Autodesk Inventor part; units mm, degrees
ref_plane "YZ Plane" through (0, 0, 0) normal (1, 0, 0) x (0, 1, 0)
ref_plane "XZ Plane" through (0, 0, 0) normal (0, 1, 0) x (-1, 0, 0)
ref_plane "XY Plane" through (0, 0, 0) normal (0, 0, 1) x (1, 0, 0)
ref_plane "Plano de trabajo1" through (0, 0, 0) normal (0, 0, 1) x (1, 0, 0)
sketch "Boceto1" plane through (0, 0, 0) normal (0, 0, 1) x (1, 0, 0)
  circle A0 centre (18.3423, 0) radius 1.2028
  circle A1 centre (3.6423, 0) radius 1.2028
  circle A2 centre (10.9923, -7.35) radius 1.2028
  circle A3 centre (10.9923, 7.35) radius 1.2028
  circle A4 centre (10.9923, 0) radius 10.9823
  circle A5 centre (10.9923, 0) radius 2.7
  circle A6 centre (10.9923, 0) radius 12.5
  line L0 (10.9923, 0) -> (22.9923, 0)
  line L1 (10.9923, 0) -> (10.9923, 12.5)
  line L2 (10.9923, 12.5) -> (22.9923, 12.5)
  line L3 (10.9923, 0) -> (10.9923, -12.5)
  line L4 (10.9923, -12.5) -> (22.9923, -12.5)
  line L5 (22.9923, -12.5) -> (22.9923, 12.5)
  point P0 (0, 0)
  dimension "d0" = 25
  dimension "d1" = 12
  dimension "d2" = 12
extrude "Extrusión1" add sketch "Boceto1" along normal blind 3 contours L0 A4 L3 A2 A5 A0 | A0 L0 A5 L1 A3 A4 | L0 L5 A6 L3 A4 | A4 L1 A6 L5 L0 | L1 A3 A5 L3 A2 A4 | A4 L3 A6 L1 | L2 L5 A6 | A6 L5 L4
sketch "Boceto2" plane through (22.9923, -12.5, 0) normal (1, 0, 0) x (0, 0, -1)
  line L0 (0, 0) -> (0, 25)
  line L1 (0, 25) -> (-3, 25)
  line L2 (-3, 0) -> (-3, 25)
  line L3 (0, 0) -> (-3, 0)
  point P0 (0, 12.5)
extrude "Extrusión2" add sketch "Boceto2" along normal blind 8
sketch "Boceto3" plane through (0, 0, 0) normal (0, 0, -1) x (-1, 0, 0)
  line L0 (-10.9923, -12.5) -> (-30.9923, -12.5)
  arc A0 (-10.9923, -12.5) -> (-10.9923, 12.5) centre (-10.9923, 0) ccw
  line L1 (-10.9923, 12.5) -> (-30.9923, 12.5)
  line L2 (-30.9923, -12.5) -> (-30.9923, 12.5)
  circle A1 centre (-10.9923, 0) radius 2.7
  circle A2 centre (-10.9923, 7.35) radius 1.2028
  circle A3 centre (-18.3423, 0) radius 1.2028
  circle A4 centre (-3.6423, 0) radius 1.2028
  circle A5 centre (-10.9923, -7.35) radius 1.2028
  line L3 (-30.9923, 12.5) -> (-27.9923, 12.5)
  line L4 (-27.9923, 12.5) -> (-27.9923, -12.5)
  line L5 (-27.9923, -12.5) -> (-30.9923, -12.5)
  line L6 (-30.9923, -12.5) -> (-30.9923, 12.5)
  point P0 (0, 0)
  dimension "d7" = 3
extrude "Extrusión3" add sketch "Boceto3" along normal blind 42 contours L0 L2 L1 L4
sketch "Boceto4" plane through (27.9923, -12.5, 0) normal (-1, 0, 0) x (0, 0, 1)
  line L0 (-42, 0) -> (-42, 25)
  line L1 (0, 25) -> (0, 0)
  line L2 (0, 25) -> (-42, 25)
  line L3 (-42, 0) -> (-42, 25)
  line L4 (0, 0) -> (-42, 0)
  line L5 (-42, 0) -> (-40, 0)
  line L6 (-40, 0) -> (-40, 25)
  line L7 (-40, 25) -> (-42, 25)
  line L8 (-42, 25) -> (-42, 0)
  point P0 (0, 12.5)
  dimension "d10" = 2
extrude "Extrusión4" add sketch "Boceto4" along normal blind 30 contours L0 L2 L6 L4
sketch "Boceto5" plane through (0, 0, -42) normal (0, 0, -1) x (-1, 0, 0)
  line L0 (24.4501, 12.6367) -> (24.5578, -12.3277)
  line L1 (-11.0672, 12.4835) -> (24.4501, 12.6367)
  arc A0 (-11.0672, 12.4835) -> (-10.9596, -12.4809) centre (-11.0134, 0.0013) ccw
  line L2 (-10.9596, -12.4809) -> (24.5578, -12.3277)
  circle A1 centre (-3.6676, 0.2495) radius 1.2028
  circle A2 centre (-11.0134, 0.0013) radius 2.7
  circle A3 centre (-10.7652, -7.3445) radius 1.2028
  circle A4 centre (-11.2616, 7.3471) radius 1.2028
  circle A5 centre (-18.3592, -0.2469) radius 1.2028
  line L3 (-30.9923, 12.5) -> (2.0077, 12.5)
  line L4 (-11.0672, 12.4835) -> (2.0077, 12.5)
  line L5 (2.0391, -12.4248) -> (2.0077, 12.5)
  line L6 (-10.9596, -12.4809) -> (2.0391, -12.4248)
  line L7 (-11.0672, 12.4835) -> (2.0077, 12.5)
  circle A6 centre (-11.0134, 0.0013) radius 12.4823
  line L8 (-10.7652, -7.3445) -> (-10.7652, -14.8497)
  line L9 (-10.7652, -14.8497) -> (6.2045, -14.8497)
  line L10 (6.2045, -14.8497) -> (6.2045, 15.7882)
  line L11 (6.2045, 15.7882) -> (-10.7652, 15.7882)
  line L12 (-10.7652, 15.7882) -> (-11.2616, 7.3471)
  point P0 (0, 0)
  point P1 (-7.2489, 12.5)
  point P2 (-10.991, 12.4836)
  point P3 (-10.9817, -12.481)
  point P4 (-10.9586, 12.5)
  point P5 (6.2045, 12.558)
  point P6 (6.2045, -12.4069)
  point P7 (-10.7652, -12.48)
  point P8 (-10.9595, 12.484)
  point P9 (-10.9595, 12.4837)
  point P10 (-10.9596, 12.4835)
  point P11 (-10.991, 12.4836)
  point P12 (-10.7652, -12.4785)
  point P13 (-11.0672, 12.4835)
extrude "Extrusión5" cut sketch "Boceto5" against normal blind 25 contours L10 L2 L5 L3 L1 | L1 L3 L12 L11 L10 | L10 L9 L8 L2 | L3 L4 L1 | L1 L12 L3 | L2 A6 L4 L5 | A3 | A4 | A1 | A2 | A5
sketch "Boceto8" plane through (10.9923, -12.5, 0) normal (0, -1, 0) x (1, 0, 0)
  line L0 (-0.2271, -40) -> (-0.2271, -42)
  line L1 (20, -42) -> (-0.2271, -42)
  line L2 (20, 3) -> (20, -42)
  line L3 (0, 3) -> (20, 3)
  line L4 (0, 0) -> (0, 3)
  line L5 (0, 0) -> (17, 0)
  line L6 (17, 0) -> (17, -40)
  line L7 (17, -40) -> (-0.2271, -40)
  line L8 (20, -42) -> (20, -19.5)
  line L9 (20, 3) -> (20, -42)
  line L10 (20, -19.5) -> (20, -23.5)
  line L11 (20, -23.5) -> (20, -15.5)
  line L12 (20, -15.5) -> (17, -15.5)
  line L13 (20, -23.5) -> (17, -23.5)
  point P0 (-10.9923, 0)
  dimension "d29" = 22.5
  dimension "d30" = 4
  dimension "d31" = 8
extrude "Extrusión8" add sketch "Boceto8" along normal blind 6 contours L6 L12 L2 L13
ref_plane "Plano de trabajo2" through (-0.8313, -11.6464, -27.56) normal (0.0048, -1, 0) x (1, 0.0048, 0)
sketch "Boceto9" plane through (30.9923, -12.5, 0) normal (1, 0, 0) x (0, 0, -1)
  line L0 (-3, 25) -> (42, 25)
  line L1 (-3, 25) -> (-3, 0)
  line L2 (-3, 0) -> (15.5, 0)
  line L3 (15.5, 0) -> (15.5, -6)
  line L4 (23.5, -6) -> (15.5, -6)
  line L5 (23.5, 0) -> (23.5, -6)
  line L6 (23.5, 0) -> (42, 0)
  line L7 (42, 25) -> (42, 0)
  line L8 (23.5, 0) -> (23.5, 25)
  line L9 (23.5, 25) -> (23.5, 31)
  line L10 (23.5, 31) -> (15.5, 31)
  line L11 (15.5, 31) -> (15.5, 25)
  point P0 (0, 12.5)
  dimension "d34" = 6
extrude "Extrusión9" add sketch "Boceto9" against normal blind 3 contours L11 L10 L9 L0
sketch "Boceto10" plane through (27.9923, -12.5, 0) normal (-1, 0, 0) x (0, 0, 1)
  line L0 (-40, 25) -> (-40, 0)
  line L1 (-23.5, 0) -> (-40, 0)
  line L2 (-23.5, 0) -> (-23.5, -6)
  line L3 (-15.5, -6) -> (-23.5, -6)
  line L4 (-15.5, 0) -> (-15.5, -6)
  line L5 (0, 0) -> (-15.5, 0)
  line L6 (0, 25) -> (0, 0)
  line L7 (0, 25) -> (-15.5, 25)
  line L8 (-15.5, 25) -> (-15.5, 31)
  line L9 (-15.5, 31) -> (-23.5, 31)
  line L10 (-23.5, 31) -> (-23.5, 25)
  line L11 (-23.5, 25) -> (-40, 25)
  line L12 (-15.5, -3) -> (-19.5, -3)
  line L13 (-19.5, -3) -> (-19.5, 28)
  circle A0 centre (-19.5, -3) radius 1.25
  circle A1 centre (-19.5, 28) radius 1.25
  point P0 (0, 12.5)
  dimension "d37" = 2.5
  dimension "d38" = 2.5
extrude "Extrusión10" cut sketch "Boceto10" against normal blind 3 contours A1 | A0 L13 L12 | L12 L13 A0
sketch "Boceto11" plane through (27.9923, -12.5, 0) normal (-1, 0, 0) x (0, 0, 1)
  line L0 (-42, 25) -> (-42, 0)
  line L1 (-42, 25) -> (-42, 12.5)
  line L2 (-42, 12.5) -> (-19.5, 12.5)
  line L3 (3, 13.7028) -> (3, 11.2972)
  line L4 (-19.5, 12.5) -> (-19.5, 25)
  point P0 (0, 12.5)
  dimension "d41" = 12.5
  dimension "d42" = 22.5
properties part number "UnionCuerpo"
Part model, mm, in its own coordinate system. A direction names the side the tool comes from. Give positions to 0.01 mm unless a question says otherwise; leave off trailing zeros. Loops run counter-clockwise (first coordinate to the right, second up) from the corner with the lowest first, then second, coordinate; pieces in that order, holes last. Notation, with made-up numbers: M 10.5,28.25 L 15.5,28.25 A15 ccw 15.5,40.25 Z; hole C -18.75,62.25 d10. An arc over 180 degrees is marked long. Return JSON: item names as keys, results as strings.
1) Pull direction Y, two halves, no side cores. Call faces 1 (the face through (27.992, 0, -20)), 2 (the face through (-1.505, -0.275, 1.479)), 3 (the face through (11.547, -6.283, 1.479)): released by +Y, released by -Y, zero draft, split by the parting line, or undercut.
Calculated:
{"face 1": "zero draft", "face 2": "split by the parting line", "face 3": "undercut"}
2) 3-axis set-ups, long thin cutter, end or side, ignore diameter. For faces 4 (the face through (11.967, -7.292, -41.014)), 5 (the face through (29, 12.5, -36)), 6 (the face through (17, 0, -40)), 7 (the face through (19.49, -0.36, 1.48)), 8 (the face through (25, 12.5, 1)): which of +Z, -Z, +X, -X, +Y, -Y reach the whole face in a straight line?
Calculated:
{"face 4": "-Z", "face 5": "-Z, +X, -X, +Y", "face 6": "-X, +Y, -Y", "face 7": "+Z", "face 8": "+Z, +X, -X, +Y"}
3) Saw through at B-B, the plane x = 23.5. List the corners of the cut face in (y, z), then the cut area to 3 significant figures.
Calculated:
{"outline": "M -12.5,-42 L 12.5,-42 L 12.5,-40 L -12.5,-40 Z; M -12.5,0 L 12.5,0 L 12.5,3 L -12.5,3 Z", "area": "125 mm2"}
4) Saw through at A-A, the plane z = -19.5. List the corners of the cut face in (x, y).
Calculated:
{"outline": "M 27.99,-18.5 L 30.99,-18.5 L 30.99,-16.75 L 27.99,-16.75 Z; M 27.99,-14.25 L 30.99,-14.25 L 30.99,14.25 L 27.99,14.25 Z; M 27.99,16.75 L 30.99,16.75 L 30.99,18.5 L 27.99,18.5 Z"}
5) Saw through at C-C, the plane y = -15.5. List the corners of the cut face in (x, z), then the cut area to 3 significant figures.
Calculated:
{"outline": "M 27.99,-23.5 L 30.99,-23.5 L 30.99,-20.75 L 27.99,-20.75 Z; M 27.99,-18.25 L 30.99,-18.25 L 30.99,-15.5 L 27.99,-15.5 Z", "area": "16.5 mm2"}
6) Drill centre lines: line 1 (Z direction, x = 14, y = 5); line 2 (Y direction, x = 29.25, z = -19.5); line 3 (Z direction, x = 29, y = 15.5). Where is each one in solid material? Low to high.
Calculated:
{"line 1": "z = -42 to -40, 0 to 3", "line 2": "y = -18.5 to -16.75, -14.25 to 14.25, 16.75 to 18.5", "line 3": "z = -23.5 to -20.75, -18.25 to -15.5"}
7) Flat gauge pins, fed straight in: pin 1 Ø15 at (x, z) = (17, -31.5) entering from -Y; pin 2 Ø2 at (x, y) = (18.36, -0.25) entering from -Z; pin 3 Ø0.9 at (x, y) = (30, -15) entering from +Z; pin 4 Ø4 at (x, z) = (27, -6) entering from +Y. Where does each tip first touch, or does it go through?
Calculated:
{"pin 1": "passes through", "pin 2": "stops at z = 0", "pin 3": "stops at z = -15.5", "pin 4": "stops at y = 12.5"}
8) Saw through at D-D, the plane x = 18. List the corners of the cut face in (y, z), then the cut area to 3 significant figures.
Calculated:
{"outline": "M -12.5,-42 L -1.39,-42 L -1.39,-40 L -12.5,-40 Z; M -12.5,0 L -1.15,0 L -1.15,3 L -12.5,3 Z; M 0.9,-42 L 12.5,-42 L 12.5,-40 L 0.9,-40 Z; M 1.15,0 L 12.5,0 L 12.5,3 L 1.15,3 Z", "area": "113 mm2"}
